from build123d import *

# Parameters (mm, degrees)
SKETCH2_R           = 2.5
BOSS_EXTRUDE1_DEPTH = 8
CHAMFER1_SIZE       = 0.5
CUT_EXTRUDE1_DEPTH  = 2.3
SKETCH8_R           = 1.782050808
CUT_EXTRUDE2_DEPTH  = 1
CUT_EXTRUDE2_TAPER  = 45


with BuildPart() as part:
    # Sketch2 → Boss-Extrude1 (new body)
    with BuildSketch(Plane(origin=(0, 0, 0), x_dir=(0, 0, -1), z_dir=(1, 0, 0))):
        Circle(SKETCH2_R)
    extrude(amount=-BOSS_EXTRUDE1_DEPTH)

    # Chamfer1
    chamfer1_edges = [part.edges().sort_by_distance(p)[0] for p in [
        (0, 0, 2.5),
    ]]
    chamfer(chamfer1_edges, length=CHAMFER1_SIZE)

    # Sketch6 → Revolve1 (revolve)
    with BuildSketch(Plane.XY):
        with BuildLine():
            Line((-9.5, 0), (-9.5, 4.161437828))
            ThreePointArc((-9.5, 4.161437828), (-8.75, 4.5), (-8, 4.161437828))
            Line((-8, 4.161437828), (-8, 0))
            Line((-8, 0), (-9.5, 0))
        make_face()
    revolve(axis=Axis((-8, 0, 0), (-1, 0, 0)))

    # Sketch7 → Cut-Extrude1 (cut)
    with BuildSketch(Plane.ZY.offset(9.5)):
        Polygon((0, 1.732050808), (-1.5, 0.866025404), (-1.5, -0.866025404), (0, -1.732050808), (1.5, -0.866025404), (1.5, 0.866025404), align=None)
    extrude(amount=-CUT_EXTRUDE1_DEPTH, mode=Mode.SUBTRACT)

    # Sketch8 → Cut-Extrude2 (cut)
    with BuildSketch(Plane.ZY.offset(9.5)):
        Circle(SKETCH8_R)
    extrude(amount=-CUT_EXTRUDE2_DEPTH, taper=CUT_EXTRUDE2_TAPER, mode=Mode.SUBTRACT)


solid = part.part
For this review, take the finished solid that the model builds, in its own axes (mm). A direction names the side the tool comes from. Round coordinates to 2 decimals unless told otherwise and drop trailing zeros. Loops run counter-clockwise (first coordinate to the right, second up) from the corner with the lowest first, then second, coordinate; pieces in that order, holes last. Notation, with made-up numbers: (5, -24.5) - (33, -24.5) arc R37 ccw to (33, 11.5) - close; hole circle Ø8 at (-39, 86). An arc over 180 degrees is marked (long way). Answer as CSV lines item,"result".
(1) Mouldability with a two-part tool opening along Z and no side actions: class faces 1 (the face through (-8.341, -1.293, -0.76)), 2 (the face through (-4.2, -2.44, 0.54)), 3 (the face through (-8.341, 1.305, -0.74)), 4 (the face through (-8, 2, 2)) as +Z half, -Z half, draft (parallel to the pull), parting line (faces both ways), or undercut.
Checked values:
face 1,"undercut"
face 2,"parting line"
face 3,"undercut"
face 4,"draft"
(2) Insertion check: P1, Ø5, axis at x = -4, z = 1, coming from the +Y side; P2, Ø4, axis at x = -5.5, y = 3, coming from the -Z side; P3, Ø1, axis at x = -6.5, z = -1.5, coming from the +Y side; P4, Ø1.4, axis at x = -8, y = 0, coming from the +Z side. Each pin has a flat end and moves straight along its axis. Give the tip position at first contact, or say it passes through.
Checked values:
P1,"stops at y = 2.5"
P2,"stops at z = -2.29"
P3,"stops at y = 2.29"
P4,"stops at z = 4.5"
(3) Tool access review of faces 5 (the face through (-9.5, -2, 0)), 6 (the face through (-8, 0, -1.5)): name each direction out of +Z, -Z, +X, -X, +Y, -Y from which nothing blocks a thin tool from reaching the whole face with its end or side.
Checked values:
face 5,"+Z, -Z, -X, +Y, -Y"
face 6,"-X"
(4) Consider section A-A on x = -4.5. Give the boundary of the cut face in (y, z).
Checked values:
outline,"circle Ø5 at (0, 0)"
(5) Wall thickness on line 1 (X direction, y = 3.5, z = -0.25); line 2 (Y direction, x = -1, z = 1.5); line 3 (Z direction, x = -8.25, y = -1): over which ranges is each line inside the solid? List them lowest first.
Checked values:
line 1,"x = -9.5 to -8"
line 2,"y = -2 to 2"
line 3,"z = -4.25 to -1.27, 1.27 to 4.25"
